Can you work these out from the model? Positions are in its coordinate system, mm. A direction names the side the tool comes from. Give positions to 0.01 mm unless a question says otherwise; leave off trailing zeros. Write each loop counter-clockwise with the first axis right and the second up, starting at its lowest first coordinate (ties: lowest second). Pieces come first, ordered by that corner, then holes. Notation, with made-up numbers: M -38.75,-20.5 L -27.75,-20.5 A15 cw -27.75,-0.5 Z; hole C 0.5,18 d6. An arc over 180 degrees is marked long. Answer as CSV lines item,"result". Start each with the question number.
```python
from build123d import *

# Parameters (mm, degrees)
F0_R          = 6.25
F1_DEPTH      = 1.5
F1_DEPTH_BACK = 1.5
F2_R          = 6.25
F2_R_2        = 1.45
F3_DEPTH      = 6
F4_R          = 6.25
F4_R_2        = 1.45
F5_DEPTH      = 6


with BuildPart() as f1:
    # F0 (on Top) → F1 (new body, two sides)
    with BuildSketch(Plane.XY) as f1_sk:
        Circle(F0_R)
    extrude(amount=F1_DEPTH)
    extrude(f1_sk.sketch, amount=-F1_DEPTH_BACK)

    # F2 (on face) → F3 (join)
    with BuildSketch(Plane.XY.offset(1.5)):
        Circle(F2_R)
        Circle(F2_R_2, mode=Mode.SUBTRACT)
    extrude(amount=F3_DEPTH)

    # F4 (on face) → F5 (join)
    with BuildSketch(Plane(origin=(0, 0, -1.5), x_dir=(1, 0, 0), z_dir=(0, 0, -1))):
        Circle(F4_R)
        Circle(F4_R_2, mode=Mode.SUBTRACT)
    extrude(amount=F5_DEPTH)


solid = f1.part
```
1) I want a section at D-D, the plane z = 0.5. Please give me the cut outline in (x, y), then the cut area to 3 significant figures.
2) Thinking about a two-plate mould opening in X: for faces 1 (the flat face through (0, 0, -1.5)), 2 (the flat face through (1.3, 1.3, -7.5)), 3 (the cylindrical face through (-1.45, -0.06, -4.46)), 4 (the cylindrical face through (5.96, -1.88, 0.11)), which applies, released by +X, released by -X, zero draft, split by the parting line, or undercut?
3) I want a section at C-C, the plane z = 2. Please give me the cut outline in (x, y), then the cut area to 3 significant figures.
4) I'm going to push flat-ended pins straight in: P1, Ø1.5, axis at x = 3, z = -2, coming from the +Y side; P2, Ø2.5, axis at x = 0, y = 0, coming from the +Z side. Where does each tip first touch, or does it pass through?
5) On a 3-axis mill with a long thin cutter (end or side, diameter ignored), from which of +Z, -Z, +X, -X, +Y, -Y can I reach the whole of each face in a straight line? I mean faces 5 (the cylindrical face through (-1.45, 0.06, 4.46)), 6 (the flat face through (1.3, -1.3, 7.5)). Say none if no direction works.
6) I want a section at A-A, the plane x = 0. Please give me the cut outline in (y, z), then the cut area to 3 significant figures.
7) I need wall thicknesses on L1, parallel to X at y = 0, z = -3.5; L2, parallel to Z at x = -0.25, y = 0.75. Which ranges of each line are inside material? Lowest first, please. Write a range as from..to.
Values found:
1,outline,"C 0,0 d12.5"
1,area,"123 mm²"
2,face 1,"undercut"
2,face 2,"zero draft"
2,face 3,"undercut"
2,face 4,"split by the parting line"
3,outline,"C 0,0 d12.5; hole C 0,0 d2.9"
3,area,"116 mm²"
4,P1,"stops at y = 5.83"
4,P2,"stops at z = 1.5"
5,face 5,"+Z"
5,face 6,"+Z, +X, -X, +Y, -Y"
6,outline,"M -6.25,-7.5 L -1.45,-7.5 L -1.45,-1.5 L 1.45,-1.5 L 1.45,-7.5 L 6.25,-7.5 L 6.25,7.5 L 1.45,7.5 L 1.45,1.5 L -1.45,1.5 L -1.45,7.5 L -6.25,7.5 Z"
6,area,"153 mm²"
7,L1,"x = -6.25..-1.45, 1.45..6.25"
7,L2,"z = -1.5..1.5"
